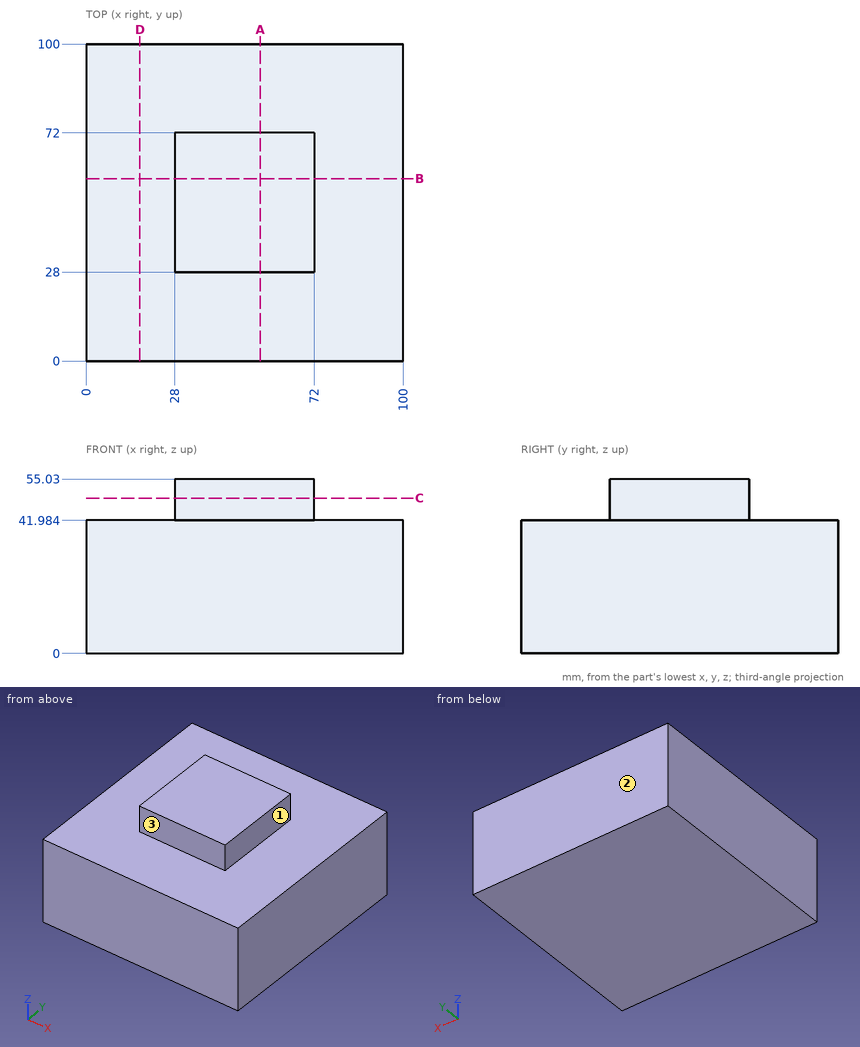
Print and shaded views of the part. All mm, measured from the part's lowest x, y and z. A direction names the side the tool comes from. Coordinates: 2 decimals unless noted, no trailing zeros. Write each loop counter-clockwise with the first axis right and the second up, starting at its lowest first coordinate (ties: lowest second). Pieces come first, ordered by that corner, then holes. Notation, with made-up numbers: M 33,-35.5 L 51,-35.5 A24 cw 51,-25.5 Z; hole C 14,-14.75 d10. An arc over 180 degrees is marked long. Return JSON: item names as keys, results as strings.
1. Probe L1, parallel to Z at x = 7.5, y = 6; L2, parallel to X at y = 28.5, z = 43. List the from-to ranges inside material, lowest first.
Determined:
{"L1": "0 to 41.98", "L2": "28 to 72"}
2. 3-axis set-ups, long thin cutter, end or side, ignore diameter. For the marked faces 1, 2 and 3: which of +Z, -Z, +X, -X, +Y, -Y reach the whole face in a straight line?
Determined:
{"face 1": "+Z, +X, +Y, -Y", "face 2": "+Z, -Z, +X, -X, +Y", "face 3": "+Z, +X, -X, -Y"}
3. Flat gauge pins, fed straight in: pin 1 Ø4 at (y, z) = (52.5, 50) entering from +X; pin 2 Ø4 at (x, z) = (60, 47) entering from -Y; pin 3 Ø4 at (x, z) = (46, 48.5) entering from +Y. Where does each tip first touch, or does it go through?
Determined:
{"pin 1": "x = 72", "pin 2": "y = 28", "pin 3": "y = 72"}
4. Saw through at C-C, the plane z = 49. Write the cut outline in (x, y).
Determined:
{"outline": "M 28,28 L 72,28 L 72,72 L 28,72 Z"}
5. Saw through at A-A, the plane x = 55. Write the cut outline in (y, z), then the cut area to 3 significant figures.
Determined:
{"outline": "M 0,0 L 100,0 L 100,41.98 L 72,41.98 L 72,55.03 L 28,55.03 L 28,41.98 L 0,41.98 Z", "area": "4,770 mm²"}
6. Saw through at D-D, the plane x = 17. Write the cut outline in (y, z), then the cut area to 3 significant figures.
Determined:
{"outline": "M 0,0 L 100,0 L 100,41.98 L 0,41.98 Z", "area": "4,200 mm²"}
